Can you work these out from the model? Positions are in its coordinate system, mm. A direction names the side the tool comes from. Round coordinates to 2 decimals unless told otherwise and drop trailing zeros. Write each loop counter-clockwise with the first axis right and the second up, starting at its lowest first coordinate (ties: lowest second). Pieces come first, ordered by that corner, then holes. Notation, with made-up numbers: M 55.25,28.5 L 95.25,28.5 A12 cw 95.25,43.5 Z; hole C 59,43 d7. An arc over 180 degrees is marked long. Answer in a Markdown table with one row per item. Add a question column.
(1) Suppose I cut it at B-B, the plane z = -3.5. Write out the boundary of the cut face in (x, y).
(2) I'm going to push flat-ended pins straight in: pin 1 (5 mm diameter, centred on x = 19, y = 28, fed in from -Z); pin 2 (5 mm diameter, centred on y = 31.5, z = 0, fed in from +X); pin 3 (2 mm diameter, centred on y = 6.5, z = 1.5, fed in from +X). Where does each tip first touch, or does it pass through?
(3) If we mould it in two halves opening along Z, with no side actions, what happens to faces 4 (the face through (-49.668, 15.986, -0.137)), 5 (the face through (48, 0, -2)), 6 (the face through (-45, 9, 0))? For each: released by +Z, released by -Z, zero draft, split by the parting line, or undercut.
(4) Suppose I cut it at C-C, the plane x = 35.5. Write out the boundary of the cut face in (y, z), then the cut area to 3 significant figures.
(5) For faces 1 (the face through (-0.52, 36.88, 1.08)), 2 (the face through (55, 9, 0)), 3 (the face through (-52, 0, -2)), which set-ups out of +Z, -Z, +X, -X, +Y, -Y let a thin tool reach every point of the face, with its end or its side?
(6) If I drill on probe 1 along Z at (x, y) = (-50, 3.75); probe 2 along X at (y, z) = (6.5, -1.5); probe 3 along X at (y, z) = (22, 4.25), over which ranges is the centre line in solid material (lowest first)?
(7) Suppose I cut it at A-A, the plane y = 6.5. Write out the boundary of the cut face in (x, z).
Autodesk Inventor part; units mm, degrees
ref_plane "bolt1_XY" through (-50, 0, 0) normal (0, 1, 0) x (1, 0, 0)
ref_plane "bolt1_YZ" through (-50, 0, 0) normal (1, 0, 0) x (0, 0, -1)
ref_plane "bolt1_ZX" through (-50, 0, 0) normal (0, 0, -1) x (0, 1, 0)
sketch "Sketch_1" plane through (0, 0, 0) normal (0, 1, 0) x (-1, 0, 0)
  circle A0 centre (50, 0) radius 5
extrude "Extrusion1" add sketch "Sketch_1" along normal blind 19
sketch "Sketch_2" plane through (0, 19, 0) normal (0, 1, 0) x (1, 0, 0)
  line L0 (-37, 5) -> (-37, -5)
  circle A0 centre (-50, 0) radius 5
revolve "Revolution1" add sketch "Sketch_2" angle 90 about axis through (-37, 19, -5) along (0, 0, -1)
sketch "Sketch_3" plane through (-37, 0, 0) normal (1, 0, 0) x (0, 0, -1)
  circle A0 centre (0, 32) radius 5
extrude "Extrusion2" add sketch "Sketch_3" along normal blind 74
sketch "Sketch_4" plane through (0, 19, 0) normal (0, 1, 0) x (1, 0, 0)
  line L0 (37, -5) -> (37, 5)
  circle A0 centre (50, 0) radius 5
revolve "Revolution2" add sketch "Sketch_4" angle 90 about axis through (37, 19, 5) along (0, 0, 1)
sketch "Sketch_5" plane through (0, 0, 0) normal (0, 1, 0) x (-1, 0, 0)
  circle A0 centre (-50, 0) radius 5
extrude "Extrusion3" add sketch "Sketch_5" along normal blind 19
sketch "Sketch_6" plane through (0, 0, 0) normal (0, 0, 1) x (1, 0, 0)
  line L0 (-50, 0) -> (-50, 16.1934)
  line L1 (-50, 16.1934) -> (-47.933, 15)
  line L2 (-47.933, 15) -> (-47.933, 0.433)
  line L3 (-47.933, 0.433) -> (-47.5, 0)
  line L4 (-47.5, 0) -> (-50, 0)
  line L5 (-50, 0) -> (-50, 16.1934)
revolve "Revolution3" cut sketch "Sketch_6" angle 360 about axis through (-50, 0, 0) along (0, -1, 0)
thread "Thread1"
sketch "Sketch_7" plane through (0, 0, 0) normal (0, 0, 1) x (1, 0, 0)
  line L0 (50, 0) -> (50, 16.1934)
  line L1 (50, 16.1934) -> (52.067, 15)
  line L2 (52.067, 15) -> (52.067, 0.433)
  line L3 (52.067, 0.433) -> (52.5, 0)
  line L4 (52.5, 0) -> (50, 0)
  line L5 (50, 0) -> (50, 16.1934)
revolve "Revolution4" cut sketch "Sketch_7" angle 360 about axis through (50, 0, 0) along (0, -1, 0)
thread "Thread2"
ref_plane "bolt1_XY" through (-50, 0, 0) normal (0, 1, 0) x (1, 0, 0)
ref_plane "bolt1_YZ" through (-50, 0, 0) normal (1, 0, 0) x (0, 0, -1)
ref_plane "bolt1_ZX" through (-50, 0, 0) normal (0, 0, -1) x (0, 1, 0)
ref_plane "bolt2_XY" through (50, 0, 0) normal (0, 1, 0) x (1, 0, 0)
ref_plane "bolt2_YZ" through (50, 0, 0) normal (1, 0, 0) x (0, 0, -1)
ref_plane "bolt2_ZX" through (50, 0, 0) normal (0, 0, -1) x (0, 1, 0)
properties part number "UWANGF_pull100-5"
Calculated:
| question | item | result |
|---|---|---|
| 1 | outline | M -53.57,0 L -46.43,0 L -46.43,19 A9.43 cw -37,28.43 L 37,28.43 A9.43 cw 46.43,19 L 46.43,0 L 53.57,0 L 53.57,19 A16.57 ccw 37,35.57 L -37,35.57 A16.57 ccw -53.57,19 Z |
| 2 | pin 1 | z = -4.77 |
| 2 | pin 2 | x = 51.97 |
| 2 | pin 3 | x = 54.97 |
| 3 | face 4 | undercut |
| 3 | face 5 | zero draft |
| 3 | face 6 | split by the parting line |
| 4 | outline | C 32,0 d10 |
| 4 | area | 78.5 mm² |
| 5 | face 1 | none |
| 5 | face 2 | -Y |
| 5 | face 3 | +Z, -Z, +X, -X, -Y |
| 6 | probe 1 | -5 to -2.07, 2.07 to 5 |
| 6 | probe 2 | -54.77 to -51.42, -48.58 to -45.23, 45.23 to 48.58, 51.42 to 54.77 |
| 6 | probe 3 | -52.34 to -46.92, 46.92 to 52.34 |
| 7 | outline | C -50,0 d10; C 50,0 d10; hole C -50,0 d4.13; hole C 50,0 d4.13 |
